from build123d import *

# Parameters (mm, degrees)
SKETCH1_R           = 14.25
SKETCH1_R_2         = 0.3
SKETCH1_R_3         = 0.7874
SKETCH1_R_4         = 8.5
BOSS_EXTRUDE1_DEPTH = 1.6


with BuildPart() as part:
    # Sketch1 → Boss-Extrude1 (new body)
    with BuildSketch(Plane(origin=(0, 0, 0), x_dir=(1, 0, 0), z_dir=(0, 1, 0))):
        with Locations(Location((0, 0, 0), (0, 0, 270))):
            Circle(SKETCH1_R)
        with Locations(Location((-11.172287143, -7.919595949, 0), (0, 0, 270))):
            Circle(SKETCH1_R_2, mode=Mode.SUBTRACT)
        with Locations(Location((-8.980256121, -8.980256121, 0), (0, 0, 270))):
            Circle(SKETCH1_R_3, mode=Mode.SUBTRACT)
        with Locations(Location((-2.3, -13.5, 0), (0, 0, 270))):
            Circle(SKETCH1_R_2, mode=Mode.SUBTRACT)
        with Locations(Location((0, -12.7, 0), (0, 0, 270))):
            Circle(SKETCH1_R_3, mode=Mode.SUBTRACT)
        with Locations(Location((7.919595949, -11.172287143, 0), (0, 0, 270))):
            Circle(SKETCH1_R_2, mode=Mode.SUBTRACT)
        with Locations(Location((8.980256121, -8.980256121, 0), (0, 0, 270))):
            Circle(SKETCH1_R_3, mode=Mode.SUBTRACT)
        with Locations(Location((13.5, -2.3, 0), (0, 0, 270))):
            Circle(SKETCH1_R_2, mode=Mode.SUBTRACT)
        with Locations(Location((12.7, 0, 0), (0, 0, 270))):
            Circle(SKETCH1_R_3, mode=Mode.SUBTRACT)
        with Locations(Location((-12.7, 0, 0), (0, 0, 270))):
            Circle(SKETCH1_R_3, mode=Mode.SUBTRACT)
        with Locations(Location((-13.5, 2.3, 0), (0, 0, 270))):
            Circle(SKETCH1_R_2, mode=Mode.SUBTRACT)
        with BuildLine():
            Line((-9.4, 4), (-9.4, -4))
            ThreePointArc((-9.4, -4), (-10, -4.6), (-10.6, -4))
            Line((-10.6, -4), (-10.6, 4))
            ThreePointArc((-10.6, 4), (-10, 4.6), (-9.4, 4))
        make_face(mode=Mode.SUBTRACT)
        with Locations(Location((-8.980256121, 8.980256121, 0), (0, 0, 270))):
            Circle(SKETCH1_R_3, mode=Mode.SUBTRACT)
        with Locations(Location((-7.919595949, 11.172287143, 0), (0, 0, 270))):
            Circle(SKETCH1_R_2, mode=Mode.SUBTRACT)
        with Locations(Location((0, 0, 0), (0, 0, 270))):
            Circle(SKETCH1_R_4, mode=Mode.SUBTRACT)
        with BuildLine():
            ThreePointArc((10.6, -4), (10, -4.6), (9.4, -4))
            Line((9.4, -4), (9.4, 4))
            ThreePointArc((9.4, 4), (10, 4.6), (10.6, 4))
            Line((10.6, 4), (10.6, -4))
        make_face(mode=Mode.SUBTRACT)
        with Locations(Location((0, 12.7, 0), (0, 0, 270))):
            Circle(SKETCH1_R_3, mode=Mode.SUBTRACT)
        with Locations(Location((2.3, 13.5, 0), (0, 0, 270))):
            Circle(SKETCH1_R_2, mode=Mode.SUBTRACT)
        with Locations(Location((8.980256121, 8.980256121, 0), (0, 0, 270))):
            Circle(SKETCH1_R_3, mode=Mode.SUBTRACT)
        with Locations(Location((11.172287143, 7.919595949, 0), (0, 0, 270))):
            Circle(SKETCH1_R_2, mode=Mode.SUBTRACT)
    extrude(amount=BOSS_EXTRUDE1_DEPTH)


solid = part.part
Here's how the part is built. I have some questions about the finished solid (model axes, mm). Round coordinates to 2 decimals unless told otherwise and drop trailing zeros. Write each loop counter-clockwise with the first axis right and the second up, starting at its lowest first coordinate (ties: lowest second). Pieces come first, ordered by that corner, then holes.
1. Suppose I cut it at D-D (z = 5). List the corners of the cut face in (x, y) for me.
2. I need wall thicknesses on L1, parallel to X at y = 1.05, z = -1.5; L2, parallel to Z at x = -9, y = 0.9; L3, parallel to X at y = 0.75, z = -9.5. Which ranges of each line are inside material? Lowest first, please.
3. Will these pins go through, and if not, where does the flat tip stop? pin 1 Ø0.9 at (x, z) = (-12.7, 0) entering from -Y; pin 2 Ø0.5 at (y, z) = (1, -0.5) entering from +X.
4. Suppose I cut it at B-B (x = 12.7). List the corners of the cut face in (y, z) for me, and give its area (3 significant figures).
5. Suppose I cut it at A-A (y = 0.4). State how many separate pieces and enclosed holes the cut face has, and give its area (3 significant figures).
6. Suppose I cut it at C-C (z = 9). List the corners of the cut face in (x, y) for me, and give its area (3 significant figures).
7. If we mould it in two halves opening along Y, with no side actions, what happens to faces 1 (the flat face through (-6.13, 0, 6.13)), 2 (the cylindrical face through (-8.45, 0.79, 8.4)), 3 (the flat face through (-6.13, 1.6, 6.13))? For each: released by +Y, released by -Y, zero draft, split by the parting line, or undercut.
Answer sheet:
1. outline: (-13.34, 0) - (-6.87, 0) - (-6.87, 1.6) - (-13.34, 1.6) - close; (6.87, 0) - (13.34, 0) - (13.34, 1.6) - (6.87, 1.6) - close
2. L1: x = -14.17 to -10.6, -9.4 to -8.37, 8.37 to 9.4, 10.6 to 14.17
2. L2: z = -11.05 to -9.77, -8.19 to 8.19, 9.77 to 11.05
2. L3: x = -10.62 to -9.57, -8.39 to 8.39, 9.57 to 10.62
3. pin 1: passes through
3. pin 2: stops at x = 14.25
4. outline: (0, -6.46) - (1.6, -6.46) - (1.6, -0.79) - (0, -0.79) - close; (0, 0.79) - (1.6, 0.79) - (1.6, 6.46) - (0, 6.46) - close
4. area: 18.2 mm2
5. separate pieces: 1
5. enclosed holes: 19
5. area: 372 mm2
6. outline: (-11.05, 0) - (-9.77, 0) - (-9.77, 1.6) - (-11.05, 1.6) - close; (-8.19, 0) - (8.19, 0) - (8.19, 1.6) - (-8.19, 1.6) - close; (9.77, 0) - (11.05, 0) - (11.05, 1.6) - (9.77, 1.6) - close
6. area: 30.3 mm2
7. face 1: released by -Y
7. face 2: zero draft
7. face 3: released by +Y
